Check sheet for the drawn part. Datum: minimum x, y, z corner. Units: mm. Give positions to 0.01 mm unless a question says otherwise; leave off trailing zeros. Loops run counter-clockwise (first coordinate to the right, second up) from the corner with the lowest first, then second, coordinate; pieces in that order, holes last.
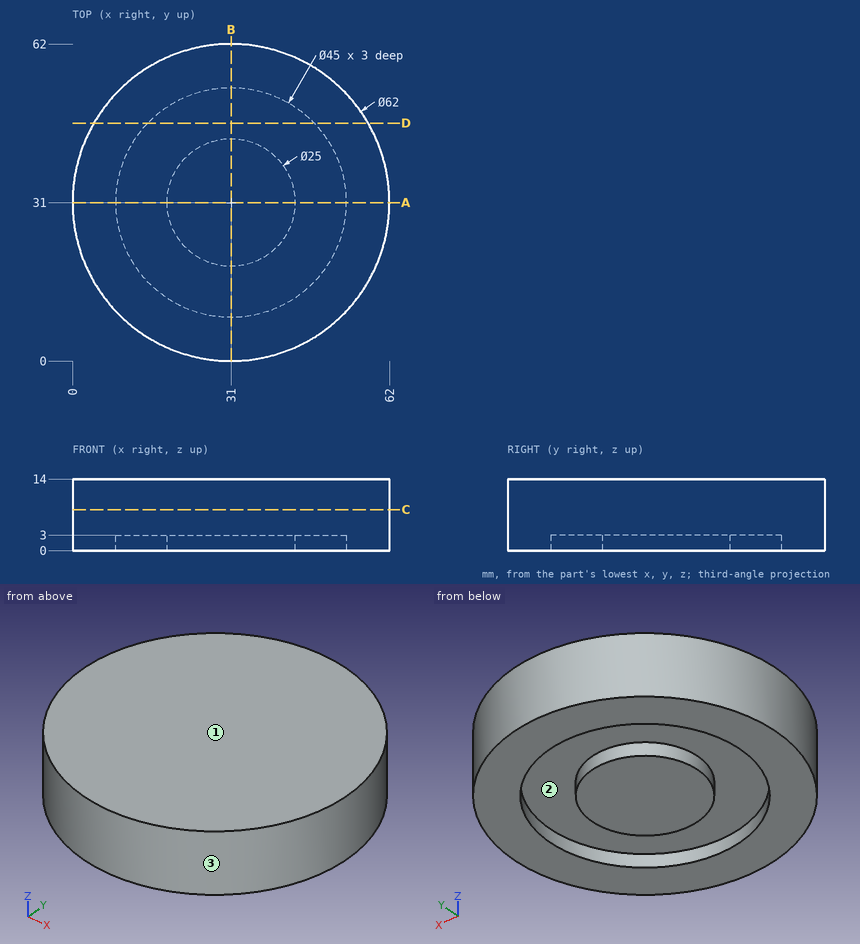
(1) Material ranges on line 1 (Y direction, x = 31, z = 1.25); line 2 (X direction, y = 27, z = 2.25); line 3 (X direction, y = 21, z = 1.5), recorded low to high.
(2) Section check D-D on y = 46.5. Record the boundary of the cut face in (x, z), plus the area to 3 significant figures.
(3) Section check A-A on y = 31. Record the boundary of the cut face in (x, z).
(4) Release check for a two-part mould opening along Y. For the marked faces 1, 2 and 3 record: pulls with the +Y half, pulls with the -Y half, needs draft (parallel to the pull), parting line crosses it, or undercut.
(5) Section check C-C on z = 8. Record the boundary of the cut face in (x, y).
(6) Gauge pin test, flat ends, axial feed: pin 1 Ø4 at (x, z) = (33.5, 8.5) entering from +Y; pin 2 Ø1.5 at (x, y) = (46.5, 14) entering from -Z; pin 3 Ø1 at (y, z) = (39, 3.5) entering from +X; pin 4 Ø1 at (x, z) = (41, 6.5) entering from -Y. Record the tip position at first contact, or that the pin passes through.
Computed values:
1. line 1: y = 0 to 8.5, 18.5 to 43.5, 53.5 to 62
1. line 2: x = 0.26 to 8.86, 19.16 to 42.84, 53.14 to 61.74
1. line 3: x = 1.66 to 10.84, 23.5 to 38.5, 51.16 to 60.34
2. outline: (4.15, 0) - (14.69, 0) - (14.69, 3) - (47.31, 3) - (47.31, 0) - (57.85, 0) - (57.85, 14) - (4.15, 14) - close
2. area: 654 mm2
3. outline: (0, 0) - (8.5, 0) - (8.5, 3) - (18.5, 3) - (18.5, 0) - (43.5, 0) - (43.5, 3) - (53.5, 3) - (53.5, 0) - (62, 0) - (62, 14) - (0, 14) - close
4. face 1: needs draft
4. face 2: undercut
4. face 3: parting line crosses it
5. outline: circle Ø62 at (31, 31)
6. pin 1: stops at y = 62
6. pin 2: stops at z = 0
6. pin 3: stops at x = 61.08
6. pin 4: stops at y = 1.49
